Study the drawing (mm; zero at the part's minimum x, y, z) and answer. A direction names the side the tool comes from. Round coordinates to 2 decimals unless told otherwise and drop trailing zeros. Write each loop counter-clockwise with the first axis right and the second up, starting at its lowest first coordinate (ties: lowest second). Pieces come first, ordered by that corner, then holes. Notation, with made-up numbers: M 63.25,-19.5 L 75.25,-19.5 A5 ccw 75.25,-13.5 Z; hole C -0.75,-15 d7. An arc over 180 degrees is marked long. Put each result on its own line as item: value. Start each with the question number.
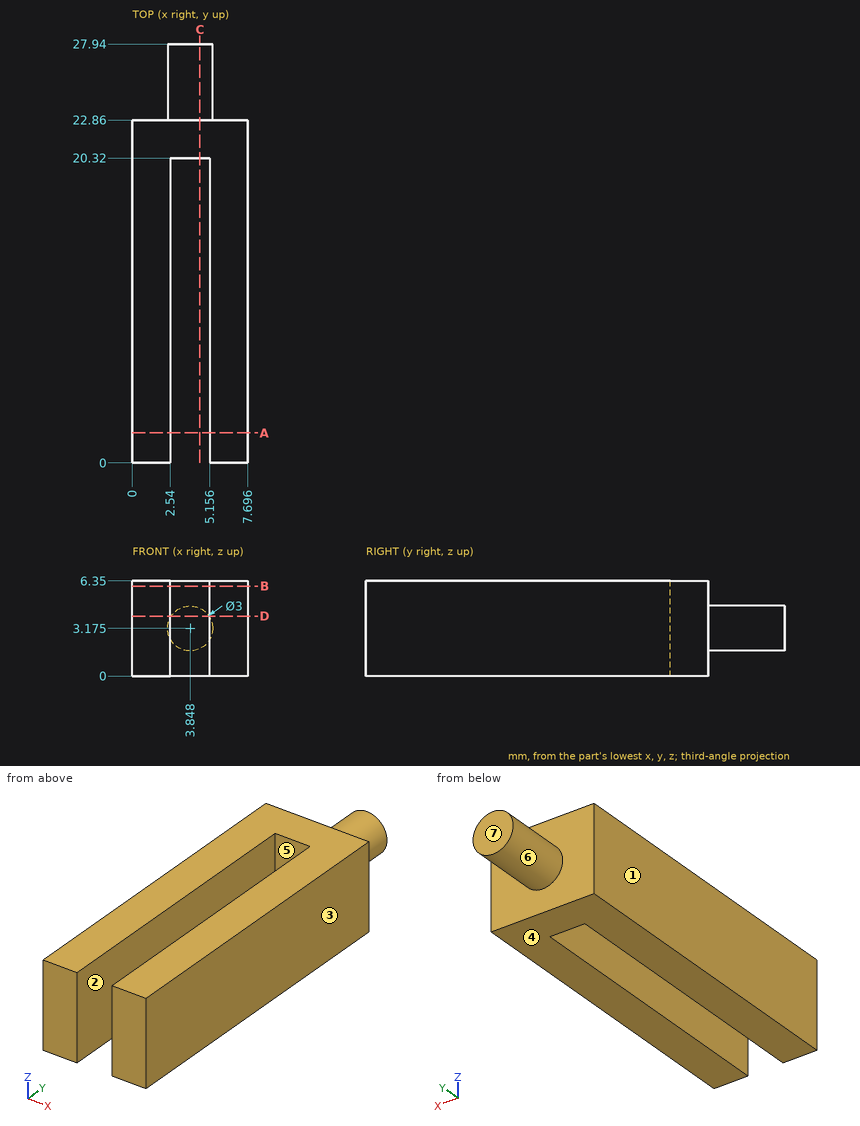
Item 1: Section D-D (z = 4) is taken. Give the vertices of the cut face in (x, y) (1 decimal).
Item 2: Section C-C (x = 4.5) is taken. Give the vertices of the cut face in (y, z).
Item 3: Consider line 1 along X through (y, z) = (15.5, 1); line 2 along Y through (x, z) = (1, 6.25); line 3 along Y through (x, z) = (3, 1.25). Determine where each line is inside the solid, lowest interval first. Write a range as [from, to].
Item 4: Determine the mould class of the marked faces 1, 2, 3 and 4 for opening direction X: released by +X, released by -X, zero draft, split by the parting line, or undercut.
Item 5: Section B-B (z = 6) is taken. Give the vertices of the cut face in (x, y), and give its area (3 significant figures).
Item 6: Section A-A (y = 2) is taken. Give the vertices of the cut face in (x, z).
Item 7: A flat-ended cylindrical pin translates along its axis: pin 1 (1 mm diameter, centred on x = 2, z = 5.5, fed in from +Y). Find the tip coordinate at first contact, or state that the pin passes through.
Item 8: Which of the six approach directions +Z, -Z, +X, -X, +Y, -Y give full straight-line access (tool end or side, diameter ignored) to the marked faces 5, 6 and 7?
Output values:
1. outline: M 0,0 L 2.5,0 L 2.5,20.3 L 5.2,20.3 L 5.2,0 L 7.7,0 L 7.7,22.9 L 5.1,22.9 L 5.1,27.9 L 2.6,27.9 L 2.6,22.9 L 0,22.9 Z
2. outline: M 20.32,0 L 22.86,0 L 22.86,1.82 L 27.94,1.82 L 27.94,4.53 L 22.86,4.53 L 22.86,6.35 L 20.32,6.35 Z
3. line 1: x = [0, 2.54], [5.16, 7.7]
3. line 2: y = [0, 22.86]
3. line 3: y = [20.32, 22.86]
4. face 1: released by -X
4. face 2: undercut
4. face 3: released by +X
4. face 4: zero draft
5. outline: M 0,0 L 2.54,0 L 2.54,20.32 L 5.16,20.32 L 5.16,0 L 7.7,0 L 7.7,22.86 L 0,22.86 Z
5. area: 123 mm^2
6. outline: M 0,0 L 2.54,0 L 2.54,6.35 L 0,6.35 Z; M 5.16,0 L 7.7,0 L 7.7,6.35 L 5.16,6.35 Z
7. pin 1: stops at y = 22.86
8. face 5: +Z, -Z, -Y
8. face 6: +Y
8. face 7: +Z, -Z, +X, -X, +Y
